```python
from build123d import *

# Parameters (mm, degrees)
F0_W      = 53.2
F0_H      = 53.2
F0_W_2    = 21.2
F0_H_2    = 21.2
F1_DEPTH  = 70
F2_W      = 8
F2_H      = 7.5
F2_H_2    = 8
F2_H_3    = 2
F4_DEPTH  = 24
F3_W      = 8
F3_H      = 23
F5_DEPTH  = 25
F2_R      = 4
F6_DEPTH  = 90
F7_W      = 8
F7_H      = 7.5
F7_H_2    = 2
F7_H_3    = 8
F8_DEPTH  = 25
F3_R      = 4
F9_DEPTH  = 100
F7_R      = 4
F10_DEPTH = 90
F11_W     = 8
F11_H     = 23
F12_DEPTH = 25
F11_R     = 4
F13_DEPTH = 90
F15_DEPTH = 25
F16_SIZE  = 1


# Not quite as in the source:
# - a feature names something its author has since deleted; it is built from what else it names


with BuildPart() as f1:
    # F0 (on Top) → F1 (new body)
    with BuildSketch(Plane.XY):
        with Locations((-29.3469955068, 26.6660622075)):
            Rectangle(F0_W, F0_H)
        with Locations((-29.3469955068, 26.6660622075)):
            Rectangle(F0_W_2, F0_H_2, mode=Mode.SUBTRACT)
    extrude(amount=F1_DEPTH)

    # F2 (on face) → F4 (cut)
    with BuildSketch(Plane(origin=(-55.9469955068, 0, 0), x_dir=(0, -1, 0), z_dir=(-1, 0, 0))):
        with Locations((-33.2660622075, 48.75)):
            Rectangle(F2_W, F2_H)
        with Locations((-33.2660622075, 56.5)):
            Rectangle(F2_W, F2_H_2)
        with Locations((-33.2660622075, 64.25)):
            Rectangle(F2_W, F2_H)
        with Locations((-33.2660622075, 69)):
            Rectangle(F2_W, F2_H_3)
        with Locations((-33.2660622075, 1)):
            Rectangle(F2_W, F2_H_3)
        with Locations((-33.2660622075, 5.75)):
            Rectangle(F2_W, F2_H)
        with Locations((-33.2660622075, 13.5)):
            Rectangle(F2_W, F2_H_2)
        with Locations((-33.2660622075, 21.25)):
            Rectangle(F2_W, F2_H)
    extrude(amount=-F4_DEPTH, mode=Mode.SUBTRACT)

    # F3 (on face) → F5 (cut)
    with BuildSketch(Plane(origin=(0, 53.2660622075, 0), x_dir=(-1, 0, 0), z_dir=(0, 1, 0))):
        with Locations((35.9469955068, 35)):
            Rectangle(F3_W, F3_H)
    extrude(amount=-F5_DEPTH, mode=Mode.SUBTRACT)

    # F2 (on face) → F6 (cut)
    with BuildSketch(Plane(origin=(-55.9469955068, 0, 0), x_dir=(0, -1, 0), z_dir=(-1, 0, 0))):
        with Locations((-47.2660622075, 35)):
            Circle(F2_R)
    extrude(amount=-F6_DEPTH, mode=Mode.SUBTRACT)

    # F7 (on face) → F8 (cut)
    with BuildSketch(Plane.YZ.offset(-2.7469955068)):
        with Locations((20.0660622075, 48.75)):
            Rectangle(F7_W, F7_H)
        with Locations((20.0660622075, 69)):
            Rectangle(F7_W, F7_H_2)
        with Locations((20.0660622075, 21.25)):
            Rectangle(F7_W, F7_H)
        with Locations((20.0660622075, 1)):
            Rectangle(F7_W, F7_H_2)
        with Locations((20.0660622075, 56.5)):
            Rectangle(F7_W, F7_H_3)
        with Locations((20.0660622075, 64.25)):
            Rectangle(F7_W, F7_H)
        with Locations((20.0660622075, 13.5)):
            Rectangle(F7_W, F7_H_3)
        with Locations((20.0660622075, 5.75)):
            Rectangle(F7_W, F7_H)
    extrude(amount=-F8_DEPTH, mode=Mode.SUBTRACT)

    # F3 (on face) → F9 (cut)
    with BuildSketch(Plane(origin=(0, 53.2660622075, 0), x_dir=(-1, 0, 0), z_dir=(0, 1, 0))):
        with Locations((49.9469955068, 56.5)):
            Circle(F3_R)
        with Locations((49.9469955068, 13.5)):
            Circle(F3_R)
    extrude(amount=-F9_DEPTH, mode=Mode.SUBTRACT)

    # F7 (on face) → F10 (cut)
    with BuildSketch(Plane.YZ.offset(-2.7469955068)):
        with Locations((6.0660622075, 35)):
            Circle(F7_R)
    extrude(amount=-F10_DEPTH, mode=Mode.SUBTRACT)

    # F11 (on face) → F12 (cut)
    with BuildSketch(Plane.XZ.offset(-0.0660622075)):
        with Locations((-22.7469955068, 35)):
            Rectangle(F11_W, F11_H)
    extrude(amount=-F12_DEPTH, mode=Mode.SUBTRACT)

    # F11 (on face) → F13 (cut)
    with BuildSketch(Plane.XZ.offset(-0.0660622075)):
        with Locations((-8.7469955068, 13.5)):
            Circle(F11_R)
        with Locations((-8.7469955068, 56.5)):
            Circle(F11_R)
    extrude(amount=-F13_DEPTH, mode=Mode.SUBTRACT)

    # F14 (on face) → F15 (cut)
    with BuildSketch(Plane(origin=(0, 53.2660622075, 0), x_dir=(-1, 0, 0), z_dir=(0, 1, 0))):
        Polygon((28.9469955068, 0), (22.1969955068, 17.5), (22.1969955068, 0), align=None)
        Polygon((27.4469955068, 35), (22.1969955068, 45.5), (22.1969955068, 24.5), align=None)
        Polygon((28.9469955068, 17.5), (24.8022586647, 17.5), (28.9469955068, 8.75), align=None)
        Polygon((28.9469955068, 52.5), (28.9469955068, 61.25), (24.8022586647, 52.5), align=None)
        Polygon((22.1969955068, 23), (24.8022586647, 17.5), (28.9469955068, 17.5), (28.9469955068, 33.5), align=None)
        Polygon((28.9469955068, 52.5), (24.8022586647, 52.5), (22.1969955068, 47), (28.9469955068, 36.5), align=None)
        Polygon((28.9469955068, 36.5), (22.1969955068, 47), (22.1969955068, 45.5), (27.4469955068, 35), (22.1969955068, 24.5), (22.1969955068, 23), (28.9469955068, 33.5), align=None)
        Polygon((24.8022586647, 17.5), (22.1969955068, 17.5), (28.9469955068, 0), (28.9469955068, 8.75), align=None)
        Polygon((24.8022586647, 52.5), (22.1969955068, 52.5), (22.1969955068, 47), align=None)
        Polygon((22.1969955068, 23), (22.1969955068, 17.5), (24.8022586647, 17.5), align=None)
        Polygon((28.9469955068, 70), (22.1969955068, 70), (22.1969955068, 52.5), align=None)
        Polygon((28.9469955068, 61.25), (28.9469955068, 70), (22.1969955068, 52.5), (24.8022586647, 52.5), align=None)
    extrude(amount=-F15_DEPTH, mode=Mode.SUBTRACT)

    # F16
    f16_edges = [f1.edges().sort_by_distance(p)[0] for p in [
        (-28.946996, 45.266062, 0),
        (-42.446996, 37.266062, 0),
        (-55.946996, 45.266062, 0),
        (-42.446996, 53.266062, 0),
        (-10.746996, 24.066062, 0),
        (-18.746996, 30.666062, 0),
        (-20.471996, 37.266062, 0),
        (-22.196996, 45.266062, 0),
        (-12.471996, 53.266062, 0),
        (-2.746996, 38.666062, 0),
        (-29.346996, 0.066062, 0),
        (-2.746996, 8.066062, 0),
        (-21.346996, 16.066062, 0),
        (-39.946996, 22.666062, 0),
        (-47.946996, 29.266062, 0),
        (-55.946996, 14.666062, 0),
        (-28.946996, 45.266062, 70),
        (-42.446996, 37.266062, 70),
        (-55.946996, 45.266062, 70),
        (-42.446996, 53.266062, 70),
        (-29.346996, 0.066062, 70),
        (-2.746996, 8.066062, 70),
        (-21.346996, 16.066062, 70),
        (-39.946996, 22.666062, 70),
        (-47.946996, 29.266062, 70),
        (-55.946996, 14.666062, 70),
        (-10.746996, 24.066062, 70),
        (-18.746996, 30.666062, 70),
        (-20.471996, 37.266062, 70),
        (-22.196996, 45.266062, 70),
        (-12.471996, 53.266062, 70),
        (-2.746996, 38.666062, 70),
    ]]
    chamfer(f16_edges, length=F16_SIZE)


solid = f1.part
```
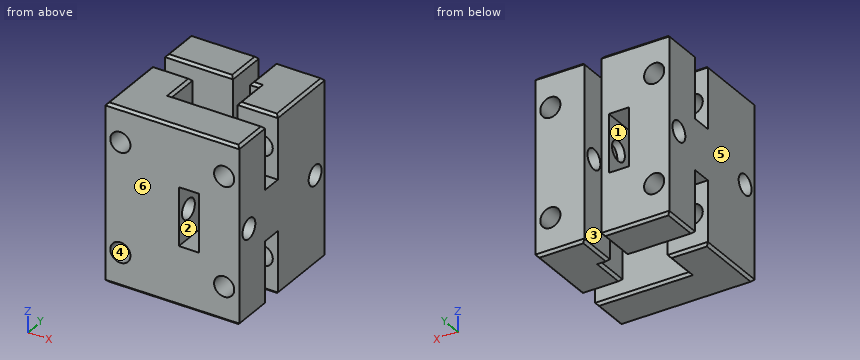
For this review, take the finished solid that the model builds, in its own axes (mm). Face numbers are marked on the shaded views. A direction names the side the tool comes from. Coordinates: 2 decimals unless noted, no trailing zeros. Loops run counter-clockwise (first coordinate to the right, second up) from the corner with the lowest first, then second, coordinate; pieces in that order, holes last. Notation, with made-up numbers: (-9, 11) - (17, 11) arc R31 ccw to (17, 46) - close; hole circle Ø1 at (78, -11). An arc over 180 degrees is marked (long way). Use one line per item in the form item = value. Start each with the question number.
1) Draft analysis for pull direction X (two halves, no side actions). For the marked faces 4, 5 and 6, state which applies: released by +X, released by -X, zero draft, split by the parting line, or undercut.
2) Take a section at C-C (z = 48). State the section outline as (x, y) points.
3) For the marked faces 1, 2 and 3, list the 3-axis set-ups (+Z, -Z, +X, -X, +Y, -Y) from which the entire face can be reached by the end or side of a thin tool; tool diameter is ignored.
4) Take a section at D-D (x = -16.5). State the section outline as (y, z) points, plus the area to 3 significant figures.
5) Take a section at B-B (z = 13.5). State how many separate pieces and enclosed holes the cut face has, plus the area to 3 significant figures.
6) To check wall thickness, follow probe 1 along X at (y, z) = (43.5, 33); probe 2 along Y at (x, z) = (-49, 19); probe 3 along Z at (x, y) = (-12, 43). State the ranges of each line that lie inside material, in increasing order. Write a range as from..to.
7) Take a section at A-A (x = -37.5). State the section outline as (y, z) points.
8) For pin 1 (17.5 mm diameter, centred on x = -52, z = 14, fed in from +Y); pin 2 (12 mm diameter, centred on x = -28.5, y = 27.5, fed in from +Z); pin 3 (6.5 mm diameter, centred on x = -12, y = 19, fed in from -Z); pin 4 (5 mm diameter, centred on x = -22, y = 35, fed in from +Z), all flat-tipped, find the tip position at first contact; note any pin that passes through.
From the geometry:
q1.face_4 = undercut
q1.face_5 = released by -X
q1.face_6 = zero draft
q2.outline = (-55.95, 0.07) - (-2.75, 0.07) - (-2.75, 16.07) - (-39.95, 16.07) - (-39.95, 29.27) - (-55.95, 29.27) - close; (-55.95, 37.27) - (-28.95, 37.27) - (-28.95, 53.27) - (-55.95, 53.27) - close; (-22.2, 37.27) - (-18.75, 37.27) - (-18.75, 24.07) - (-2.75, 24.07) - (-2.75, 53.27) - (-22.2, 53.27) - close
q3.face_1 = +Y
q3.face_2 = +Y, -Y
q3.face_3 = +Z, -Z, +Y
q4.outline = (0.07, 1) - (1.07, 0) - (15.07, 0) - (16.07, 1) - (16.07, 25) - (24.07, 25) - (24.07, 1) - (25.07, 0) - (52.27, 0) - (53.27, 1) - (53.27, 69) - (52.27, 70) - (25.07, 70) - (24.07, 69) - (24.07, 45) - (16.07, 45) - (16.07, 69) - (15.07, 70) - (1.07, 70) - (0.07, 69) - close; hole circle Ø8 at (6.07, 35); hole circle Ø8 at (47.27, 35)
q4.area = 3,220 mm2
q5.separate_pieces = 7
q5.enclosed_holes = 0
q5.area = 1,290 mm2
q6.probe_1 = -55.95..-39.95, -31.95..-28.95, -22.2..-2.75
q6.probe_2 = 0.07..29.27, 37.27..53.27
q6.probe_3 = 0..11.17, 15.83..54.17, 58.83..70
q7.outline = (0.07, 1) - (1.07, 0) - (15.07, 0) - (16.07, 1) - (16.07, 69) - (15.07, 70) - (1.07, 70) - (0.07, 69) - close; (37.27, 1) - (38.27, 0) - (52.27, 0) - (53.27, 1) - (53.27, 23.5) - (37.27, 23.5) - close; (37.27, 46.5) - (53.27, 46.5) - (53.27, 69) - (52.27, 70) - (38.27, 70) - (37.27, 69) - close; hole circle Ø8 at (6.07, 35)
q8.pin_1 = 53.27
q8.pin_2 = through
q8.pin_3 = 0.68
q8.pin_4 = 69.23
